from build123d import *

# Parameters (mm, degrees)
EXTRUDE_1_DEPTH     = 2
EXTRUDE_2_DEPTH     = 8.900017028
EXTRUDE_3_DEPTH     = 8.900017028
CUT_EXTRUDE_1_DEPTH = 7.900017028
CUT_EXTRUDE_2_DEPTH = 7.900017028
SKETCH_7_R          = 4.75
EXTRUDE_4_DEPTH     = 8.9000184
SKETCH_8_R          = 4.25
CUT_EXTRUDE_3_DEPTH = 7.9000184
SKETCH_9_R          = 3.4
CUT_EXTRUDE_4_DEPTH = 50.92850157
SKETCH_10_R         = 3.55
CUT_EXTRUDE_5_DEPTH = 50.928501787
CUT_EXTRUDE_6_DEPTH = 50.92850157
EXTRUDE_5_DEPTH     = 2
SKETCH_13_R         = 3
EXTRUDE_6_DEPTH     = 3
SKETCH_14_R         = 1.6
CUT_EXTRUDE_7_DEPTH = 55.349287024
SKETCH_15_R         = 1.75
CUT_EXTRUDE_8_DEPTH = 3


with BuildPart() as part:
    # Эскиз1 → Бобышка-Вытянуть1 (new body)
    with BuildSketch(Plane(origin=(0, 0, 0), x_dir=(1, 0, 0), z_dir=(0, 1, 0))):
        with BuildLine():
            Line((35, -27.15), (-22, -27.15))
            ThreePointArc((-22, -27.15), (-26.348706704, -25.348706704), (-28.15, -21))
            Line((-28.15, -21), (-28.15, 9.9))
            ThreePointArc((-28.15, 9.9), (-26.348706704, 14.248706704), (-22, 16.05))
            Line((-22, 16.05), (-10, 16.05))
            ThreePointArc((-10, 16.05), (-5.651293296, 14.248706704), (-3.85, 9.9))
            Line((-3.85, 9.9), (-3.85, 0))
            ThreePointArc((-3.85, 0), (-2.722361108, -2.722361108), (0, -3.85))
            Line((0, -3.85), (35, -3.85))
            ThreePointArc((35, -3.85), (39.348706704, -5.651293296), (41.15, -10))
            Line((41.15, -10), (41.15, -21))
            ThreePointArc((41.15, -21), (39.348706704, -25.348706704), (35, -27.15))
        make_face()
    extrude(amount=EXTRUDE_1_DEPTH)

    # Эскиз2 → Бобышка-Вытянуть2 (add)
    with BuildSketch(Plane(origin=(0, 2, 0), x_dir=(1, 0, 0), z_dir=(0, 1, 0))):
        with BuildLine():
            Line((-10.7, -21.5), (25.6, -21.5))
            ThreePointArc((25.6, -21.5), (31.6, -15.5), (25.6, -9.5))
            Line((25.6, -9.5), (-10.7, -9.5))
            ThreePointArc((-10.7, -9.5), (-16.7, -15.5), (-10.7, -21.5))
        make_face()
    extrude(amount=-EXTRUDE_2_DEPTH)

    # Эскиз3 → Бобышка-Вытянуть3 (add)
    with BuildSketch(Plane(origin=(0, 2, 0), x_dir=(1, 0, 0), z_dir=(0, 1, 0))):
        with BuildLine():
            Line((-26.75, -19.2), (-18.75, -19.2))
            ThreePointArc((-18.75, -19.2), (-16.982233047, -18.467766953), (-16.25, -16.7))
            Line((-16.25, -16.7), (-16.25, -11.2))
            ThreePointArc((-16.25, -11.2), (-16.982233047, -9.432233047), (-18.75, -8.7))
            Line((-18.75, -8.7), (-26.75, -8.7))
            ThreePointArc((-26.75, -8.7), (-28.517766953, -9.432233047), (-29.25, -11.2))
            Line((-29.25, -11.2), (-29.25, -16.7))
            ThreePointArc((-29.25, -16.7), (-28.517766953, -18.467766953), (-26.75, -19.2))
        make_face()
    extrude(amount=-EXTRUDE_3_DEPTH)

    # Эскиз5 → Вырез-Вытянуть1 (cut)
    with BuildSketch(Plane(origin=(0, 2, 0), x_dir=(1, 0, 0), z_dir=(0, 1, 0))):
        with BuildLine():
            Line((25.6, -10.5), (-10.7, -10.5))
            ThreePointArc((-10.7, -10.5), (-15.7, -15.5), (-10.7, -20.5))
            Line((-10.7, -20.5), (25.6, -20.5))
            ThreePointArc((25.6, -20.5), (30.6, -15.5), (25.6, -10.5))
        make_face()
    extrude(amount=-CUT_EXTRUDE_1_DEPTH, mode=Mode.SUBTRACT)

    # Эскиз6 → Вырез-Вытянуть2 (cut)
    with BuildSketch(Plane(origin=(0, 2, 0), x_dir=(1, 0, 0), z_dir=(0, 1, 0))):
        with BuildLine():
            Line((-17.25, -16.7), (-17.25, -11.2))
            ThreePointArc((-17.25, -11.2), (-17.689339828, -10.139339828), (-18.75, -9.7))
            Line((-18.75, -9.7), (-26.75, -9.7))
            ThreePointArc((-26.75, -9.7), (-27.810660172, -10.139339828), (-28.25, -11.2))
            Line((-28.25, -11.2), (-28.25, -16.7))
            ThreePointArc((-28.25, -16.7), (-27.810660172, -17.760660172), (-26.75, -18.2))
            Line((-26.75, -18.2), (-18.75, -18.2))
            ThreePointArc((-18.75, -18.2), (-17.689339828, -17.760660172), (-17.25, -16.7))
        make_face()
    extrude(amount=-CUT_EXTRUDE_2_DEPTH, mode=Mode.SUBTRACT)

    # Эскиз7 → Бобышка-Вытянуть4 (add)
    with BuildSketch(Plane(origin=(0, 2, 0), x_dir=(1, 0, 0), z_dir=(0, 1, 0))):
        with Locations(Location((-20, 8.9, 0), (0, 0, 270))):
            Circle(SKETCH_7_R)
    extrude(amount=-EXTRUDE_4_DEPTH)

    # Эскиз8 → Вырез-Вытянуть3 (cut)
    with BuildSketch(Plane(origin=(0, 2, 0), x_dir=(1, 0, 0), z_dir=(0, 1, 0))):
        with Locations(Location((-20, 8.9, 0), (0, 0, 270))):
            Circle(SKETCH_8_R)
    extrude(amount=-CUT_EXTRUDE_3_DEPTH, mode=Mode.SUBTRACT)

    # Эскиз9 → Вырез-Вытянуть4 (cut, through all)
    with BuildSketch(Plane(origin=(0, -5.900017028, 0), x_dir=(1, 0, 0), z_dir=(0, 1, 0))):
        with Locations(Location((-10.7, -15.5, 0), (0, 0, 270))):
            Circle(SKETCH_9_R)
        with Locations(Location((1.4, -15.5, 0), (0, 0, 270))):
            Circle(SKETCH_9_R)
        with Locations(Location((13.5, -15.5, 0), (0, 0, 270))):
            Circle(SKETCH_9_R)
        with Locations(Location((25.6, -15.5, 0), (0, 0, 270))):
            Circle(SKETCH_9_R)
    extrude(amount=-CUT_EXTRUDE_4_DEPTH, mode=Mode.SUBTRACT)

    # Эскиз10 → Вырез-Вытянуть5 (cut, through all)
    with BuildSketch(Plane(origin=(0, -5.9000184, 0), x_dir=(1, 0, 0), z_dir=(0, 1, 0))):
        with Locations(Location((-20, 8.9, 0), (0, 0, 180))):
            Circle(SKETCH_10_R)
    extrude(amount=-CUT_EXTRUDE_5_DEPTH, mode=Mode.SUBTRACT)

    # Эскиз11 → Вырез-Вытянуть6 (cut, through all)
    with BuildSketch(Plane(origin=(0, -5.900017028, 0), x_dir=(1, 0, 0), z_dir=(0, 1, 0))):
        with BuildLine():
            Line((-27, -13.851263122), (-27, -15.6))
            ThreePointArc((-27, -15.6), (-26.794974747, -16.094974747), (-26.3, -16.3))
            Line((-26.3, -16.3), (-19.2, -16.3))
            ThreePointArc((-19.2, -16.3), (-18.705025253, -16.094974747), (-18.5, -15.6))
            Line((-18.5, -15.6), (-18.5, -13.851263122))
            ThreePointArc((-18.5, -13.851263122), (-18.543563814, -13.608175619), (-18.668832955, -13.395344741))
            Line((-18.668832955, -13.395344741), (-19.015, -12.992043329))
            Line((-19.015, -12.992043329), (-19.015, -12.3))
            ThreePointArc((-19.015, -12.3), (-19.220025253, -11.805025253), (-19.715, -11.6))
            Line((-19.715, -11.6), (-25.785, -11.6))
            ThreePointArc((-25.785, -11.6), (-26.279974747, -11.805025253), (-26.485, -12.3))
            Line((-26.485, -12.3), (-26.485, -12.992043329))
            Line((-26.485, -12.992043329), (-26.831167045, -13.395344741))
            ThreePointArc((-26.831167045, -13.395344741), (-26.956436186, -13.608175619), (-27, -13.851263122))
        make_face()
    extrude(amount=-CUT_EXTRUDE_6_DEPTH, mode=Mode.SUBTRACT)

    # Эскиз12 → Бобышка-Вытянуть5 (add)
    with BuildSketch(Plane.XZ):
        with BuildLine():
            Line((1.5, 27.15), (11.5, 27.15))
            Line((11.5, 27.15), (11.5, 32.65))
            ThreePointArc((11.5, 32.65), (10.767766953, 34.417766953), (9, 35.15))
            Line((9, 35.15), (4, 35.15))
            ThreePointArc((4, 35.15), (2.232233047, 34.417766953), (1.5, 32.65))
            Line((1.5, 32.65), (1.5, 27.15))
        make_face()
    extrude(amount=-EXTRUDE_5_DEPTH)

    # Эскиз13 → Бобышка-Вытянуть6 (add)
    with BuildSketch(Plane.XZ):
        with Locations(Location((6.5, 31.15, 0), (0, 0, 90))):
            Circle(SKETCH_13_R)
    extrude(amount=EXTRUDE_6_DEPTH)

    # Эскиз14 → Вырез-Вытянуть7 (cut, through all)
    with BuildSketch(Plane.XZ.offset(3)):
        with Locations(Location((6.5, 31.15, 0), (0, 0, 270))):
            Circle(SKETCH_14_R)
    extrude(amount=-CUT_EXTRUDE_7_DEPTH, mode=Mode.SUBTRACT)

    # Эскиз15 → Вырез-Вытянуть8 (cut)
    with BuildSketch(Plane.XZ.offset(3)):
        with Locations(Location((6.5, 31.15, 0), (0, 0, 270))):
            Circle(SKETCH_15_R)
    extrude(amount=-CUT_EXTRUDE_8_DEPTH, mode=Mode.SUBTRACT)


solid = part.part
Work out the finished part from the listing and answer in its coordinate system (mm). A direction names the side the tool comes from. Coordinates: 2 decimals unless noted, no trailing zeros. Write each loop counter-clockwise with the first axis right and the second up, starting at its lowest first coordinate (ties: lowest second). Pieces come first, ordered by that corner, then holes. Notation, with made-up numbers: (-1, 36) - (30, 36) arc R14 cw to (30, 61) - close; hole circle Ø2 at (5, 5.5). An arc over 180 degrees is marked (long way). One line per question, with ' | ' between items.
1) For faces 1 (the face through (-28.15, 1, 20)), 2 (the face through (-23, -2, 9.7)), 3 (the face through (8, -3, 9.5)), 4 (the face through (-16.963, -3.402, 9.452)), 5 (the face through (-23, -3, 8.7)), determine the directions among +Z, -Z, +X, -X, +Y, -Y from which every point of the face is accessible in a straight line to the end or side of a thin tool.
Checks:
face 1: +Z, -X, +Y, -Y | face 2: +Y | face 3: -Z, +X, -Y | face 4: -Y | face 5: +X, -X, -Y
2) Consider probe 1 along X at (y, z) = (-6.2, 15.5); probe 2 along Z at (x, y) = (25, -2.5); probe 3 along Z at (x, y) = (-21, -1.25). Determine where each line is inside the solid, lowest interval first. Write a range as [from, to].
Checks:
probe 1: [-29.25, -27], [-18.5, -14.1], [-7.3, -2], [4.8, 10.1], [16.9, 22.2], [29, 31.6] | probe 2: [9.5, 10.5], [20.5, 21.5] | probe 3: [-13.54, -13.03], [-4.77, -4.26], [8.7, 9.7], [18.2, 19.2]
3) Find section C-C, the plane z = -8. Determine the outline of the cut face in (x, y).
Checks:
outline: (-28.15, 0) - (-24.66, 0) - (-24.66, -6.9) - (-23.43, -6.9) - (-23.43, -5.9) - (-24.15, -5.9) - (-24.15, 2) - (-28.15, 2) - close; (-16.57, -6.9) - (-15.34, -6.9) - (-15.34, 0) - (-3.85, 0) - (-3.85, 2) - (-15.85, 2) - (-15.85, -5.9) - (-16.57, -5.9) - close
4) Find section B-B, the plane x = 13.5. Determine the outline of the cut face in (y, z).
Checks:
outline: (-6.9, 9.5) - (0, 9.5) - (0, 3.85) - (2, 3.85) - (2, 10.5) - (-5.9, 10.5) - (-5.9, 12.1) - (-6.9, 12.1) - close; (-6.9, 18.9) - (-5.9, 18.9) - (-5.9, 20.5) - (2, 20.5) - (2, 27.15) - (0, 27.15) - (0, 21.5) - (-6.9, 21.5) - close
5) The mould has two halves that part along X. Classify faces 6 (the face through (-16.79, -3.4, -12.4)), 7 (the face through (-17.68, -1.89, 10.15)), 8 (the face through (39.396, 0.986, 25.301)): +X half, -X half, draft (parallel to the pull), parting line (faces both ways), or undercut.
Checks:
face 6: parting line | face 7: undercut | face 8: +X half
6) Flat-ended cylindrical pins translate along their axes: P1, Ø1, axis at x = 7, z = 30.5, coming from the -Y side; P2, Ø1.5, axis at x = 20.5, y = 0, coming from the +Z side; P3, Ø0.8, axis at y = -6.5, z = 15, coming from the +X side; P4, Ø1.6, axis at y = 1.5, z = -7.5, coming from the +X side. Find the tip coordinate at first contact, or state that the pin passes through.
Checks:
P1: through | P2: z = 27.15 | P3: x = 31.6 | P4: x = -3.85
7) Find section A-A, the plane y = -4.5. Determine the outline of the cut face in (x, z), and give its area (3 significant figures).
Checks:
outline: (-29.25, 11.2) arc R2.5 ccw to (-26.75, 8.7) - (-18.75, 8.7) arc R2.5 ccw to (-16.25, 11.2) - (-16.25, 13.22) arc R6 ccw to (-10.7, 9.5) - (25.6, 9.5) arc R6 ccw to (25.6, 21.5) - (-10.7, 21.5) arc R6 ccw to (-16.37, 17.46) arc R2.5 ccw to (-18.75, 19.2) - (-26.75, 19.2) arc R2.5 ccw to (-29.25, 16.7) - close; circle Ø9.5 at (-20, -8.9); hole (-28.25, 11.2) arc R1.5 ccw to (-26.75, 9.7) - (-18.75, 9.7) arc R1.5 ccw to (-17.25, 11.2) - (-17.25, 16.7) arc R1.5 ccw to (-18.75, 18.2) - (-26.75, 18.2) arc R1.5 ccw to (-28.25, 16.7) - close; hole circle Ø8.5 at (-20, -8.9); hole (-10.7, 10.5) - (25.6, 10.5) arc R5 ccw to (25.6, 20.5) - (-10.7, 20.5) arc R5 ccw to start | area: 160 mm2
